```python
from build123d import *

# Parameters (mm, degrees)
F0_R     = 25
F1_DEPTH = 14
F2_R     = 5
F3_DEPTH = 28
F4_R     = 25
F5_DEPTH = 14
F6_SIZE  = 0.5


with BuildPart() as f1:
    # F0 (on Right) → F1 (new body)
    with BuildSketch(Plane.YZ):
        Circle(F0_R)
    extrude(amount=F1_DEPTH)

    # F2 (on face) → F3 (join)
    with BuildSketch(Plane(origin=(0, 0, 0), x_dir=(0, -1, 0), z_dir=(-1, 0, 0))):
        Circle(F2_R)
    extrude(amount=F3_DEPTH)

    # F4 (on face) → F5 (join)
    with BuildSketch(Plane(origin=(-28, 0, 0), x_dir=(0, -1, 0), z_dir=(-1, 0, 0))):
        Circle(F4_R)
    extrude(amount=F5_DEPTH)

    # F6
    f6_edges = [f1.edges().sort_by_distance(p)[0] for p in [
        (14, -25, 0),
        (0, -25, 0),
        (-35, -25, 0),
        (-28, 25, 0),
        (-42, 25, 0),
    ]]
    chamfer(f6_edges, length=F6_SIZE)


solid = f1.part
```
The listing builds one solid part. Answer for the finished solid, in the listing's coordinates (mm). Give positions to 0.01 mm unless a question says otherwise; leave off trailing zeros. Order: outer loops, then holes, each group sorted by start corner. A loop starts at its lowest first (then second) coordinate and runs counter-clockwise, first axis right, second up. Notation, with made-up numbers: (-23, 24.25) -> (-9, 24.25) arc R31 ccw to (-9, 61.25) -> close; hole circle Ø6 at (22, 88.5). An arc over 180 degrees is marked (long way). Answer as a JSON object with one key per item and string values. Group by question number.
Item 1: The part is cut by section D-D on x = -36. Write down the section's boundary in (y, z).
Item 2: The part is cut by section A-A on z = 0. Write down the section's boundary in (x, y), and give its area (3 significant figures).
Item 3: Flat-ended cylindrical pins translate along their axes: pin 1 (3 mm diameter, centred on x = -29, z = -18.5, fed in from +Y); pin 2 (6 mm diameter, centred on x = 1.5, y = 17.5, fed in from +Z); pin 3 (5 mm diameter, centred on x = -17.5, y = 1.5, fed in from +Z). Find the tip coordinate at first contact, or state that the pin passes through.
Item 4: Consider L1, parallel to X at y = 9, z = 12.5; L2, parallel to Y at x = 11.5, z = 15; L3, parallel to Z at x = 6.5, y = -7. Determine where each line is inside the solid, lowest interval first. Write a range as from..to.
Item 5: The part is cut by section C-C on x = -22. Write down the section's boundary in (y, z).
Item 6: Determine the mould class of faces 1 (the cylindrical face through (6.909, 23.846, 7.509)), 2 (the flat face through (-42, 0, 0)), 3 (the cylindrical face through (-13.8, 1.08, -4.88)) for opening direction X: pulls with the +X half, pulls with the -X half, needs draft (parallel to the pull), parting line crosses it, or undercut.
Result set:
{
 "1": {"outline": "circle Ø50 at (0, 0)"},
 "2": {"outline": "(-42, -24.5) -> (-41.5, -25) -> (-28.5, -25) -> (-28, -24.5) -> (-28, -5) -> (0, -5) -> (0, -24.5) -> (0.5, -25) -> (13.5, -25) -> (14, -24.5) -> (14, 24.5) -> (13.5, 25) -> (0.5, 25) -> (0, 24.5) -> (0, 5) -> (-28, 5) -> (-28, 24.5) -> (-28.5, 25) -> (-41.5, 25) -> (-42, 24.5) -> close", "area": "1,680 mm²"},
 "3": {"pin 1": "y = 18.33", "pin 2": "z = 20.37", "pin 3": "z = 5"},
 "4": {"L1": "-42..-28, 0..14", "L2": "-20..20", "L3": "-24..24"},
 "5": {"outline": "circle Ø10 at (0, 0)"},
 "6": {"face 1": "needs draft", "face 2": "pulls with the -X half", "face 3": "undercut"}
}
